```python
from build123d import *

# Parameters (mm, degrees)
SKETCH2_R               = 3
CUT_EXTRUDE2_DEPTH      = 21
CUT_EXTRUDE2_DEPTH_BACK = 1
SKETCH3_R               = 5.5
CUT_EXTRUDE3_DEPTH      = 11
CUT_EXTRUDE4_REACH      = 16.5
SKETCH4_R               = 1.25
CHAMFER1_SIZE           = 1


with BuildPart() as part:
    # Sketch1 → Revolve1 (revolve)
    with BuildSketch(Plane.XY):
        Polygon((27.5, 0), (27.5, 20), (25, 20), (25, 13.5), (12, 13.5), (12, 20), (0, 20), (0, 5.5), (22.4, 5.5), (22.4, 0), align=None)
    revolve(axis=Axis((0, -626.687351978, 0), (0, 1, 0)))

    # Sketch2 → Cut-Extrude2 (cut, two sides)
    with BuildSketch(Plane(origin=(0, 0, 0), x_dir=(1, 0, 0), z_dir=(0, 1, 0))) as cut_extrude2_sk:
        with Locations((-14.142135624, 14.142135624)):
            Circle(SKETCH2_R)
        with Locations((14.142135624, 14.142135624)):
            Circle(SKETCH2_R)
        with Locations((14.142135624, -14.142135624)):
            Circle(SKETCH2_R)
        with Locations((-14.142135624, -14.142135624)):
            Circle(SKETCH2_R)
    extrude(amount=CUT_EXTRUDE2_DEPTH, mode=Mode.SUBTRACT)
    extrude(cut_extrude2_sk.sketch, amount=-CUT_EXTRUDE2_DEPTH_BACK, mode=Mode.SUBTRACT)

    # Sketch3 → Cut-Extrude3 (cut)
    with BuildSketch(Plane.XZ):
        with Locations((-14.142135624, 14.142135624)):
            Circle(SKETCH3_R)
        with Locations((14.142135624, 14.142135624)):
            Circle(SKETCH3_R)
        with Locations((14.142135624, -14.142135624)):
            Circle(SKETCH3_R)
        with Locations((-14.142135624, -14.142135624)):
            Circle(SKETCH3_R)
    extrude(amount=-CUT_EXTRUDE3_DEPTH, mode=Mode.SUBTRACT)

    # Sketch4 → Cut-Extrude4 (cut, up to next)
    with BuildSketch(Plane.XZ.offset(-5.5), mode=Mode.PRIVATE) as cut_extrude4_sk1:
        with Locations((0, 20)):
            Circle(SKETCH4_R)
    cut_extrude4_tool1 = extrude(cut_extrude4_sk1.sketch, amount=-CUT_EXTRUDE4_REACH, mode=Mode.PRIVATE) & part.part
    add(cut_extrude4_tool1.solids().sort_by_distance((0, 5.5, 20))[0], mode=Mode.SUBTRACT)
    # Sketch4 → Cut-Extrude4 (cut, up to next)
    with BuildSketch(Plane.XZ.offset(-5.5), mode=Mode.PRIVATE) as cut_extrude4_sk2:
        with Locations((-20, 0)):
            Circle(SKETCH4_R)
    cut_extrude4_tool2 = extrude(cut_extrude4_sk2.sketch, amount=-CUT_EXTRUDE4_REACH, mode=Mode.PRIVATE) & part.part
    add(cut_extrude4_tool2.solids().sort_by_distance((-20, 5.5, 0))[0], mode=Mode.SUBTRACT)
    # Sketch4 → Cut-Extrude4 (cut, up to next)
    with BuildSketch(Plane.XZ.offset(-5.5), mode=Mode.PRIVATE) as cut_extrude4_sk3:
        with Locations((0, -20)):
            Circle(SKETCH4_R)
    cut_extrude4_tool3 = extrude(cut_extrude4_sk3.sketch, amount=-CUT_EXTRUDE4_REACH, mode=Mode.PRIVATE) & part.part
    add(cut_extrude4_tool3.solids().sort_by_distance((0, 5.5, -20))[0], mode=Mode.SUBTRACT)
    # Sketch4 → Cut-Extrude4 (cut, up to next)
    with BuildSketch(Plane.XZ.offset(-5.5), mode=Mode.PRIVATE) as cut_extrude4_sk4:
        with Locations((20, 0)):
            Circle(SKETCH4_R)
    cut_extrude4_tool4 = extrude(cut_extrude4_sk4.sketch, amount=-CUT_EXTRUDE4_REACH, mode=Mode.PRIVATE) & part.part
    add(cut_extrude4_tool4.solids().sort_by_distance((20, 5.5, 0))[0], mode=Mode.SUBTRACT)

    # Chamfer1
    chamfer1_edges = [part.edges().sort_by_distance(p)[0] for p in [
        (-12, 20, 0),
        (-27.5, 0, 0),
        (-27.5, 20, 0),
    ]]
    chamfer(chamfer1_edges, length=CHAMFER1_SIZE)


solid = part.part
```
Geometry: final body of the model. Coordinates: model frame, mm. A direction names the side the tool comes from. Round coordinates to 2 decimals unless told otherwise and drop trailing zeros. Write each loop counter-clockwise with the first axis right and the second up, starting at its lowest first coordinate (ties: lowest second). Pieces come first, ordered by that corner, then holes. Notation, with made-up numbers: (-14, -33.5) -> (-9, -33.5) arc R7 ccw to (-9, -22.5) -> close; hole circle Ø4 at (12.5, 34). An arc over 180 degrees is marked (long way). Use CSV: the item, a comma, the result in double quotes. Start each with the question number.
Q1. Line query: L1, parallel to X at y = 18.5, z = 0; L2, parallel to X at y = 16.5, z = -9; L3, parallel to Z at x = -8, y = 19. Output: solid intervals per line, ascending.
Q2. Section A-A (x = 0). Give the number of separate pieces and of enclosed holes in the cut face, plus the area to 3 significant figures.
Q3. Section C-C (y = 18). Return loops of the section in (x, z), plus the area to 3 significant figures.
Q4. Reachability of faces 1 (the face through (-18.845, 9.444, -0.479)), 2 (the face through (-18.5, 6.6, -17.5)) from +Z, -Z, +X, -X, +Y, -Y: full face, straight path, thin tool, end or side. Return the list, or none.
Q5. Pull-direction query (Z, two-part tool) for faces 3 (the face through (20, 20, -16)), 4 (the face through (-5.961, 10.126, 26.846)), 5 (the face through (-6, 13.5, 11)); classes: pulls with the +Z half, pulls with the -Z half, needs draft (parallel to the pull), parting line crosses it, or undercut.
Q6. Section D-D (y = 3). Return loops of the section in (x, z).
Q7. First-contact query: pin 1 Ø5.5 at (x, z) = (16.5, -13.5) entering from -Y; pin 2 Ø2 at (x, z) = (15.5, 4.5) entering from -Y; pin 3 Ø4 at (x, z) = (0, -20) entering from +Y. Flat tips, straight axial feed; report the tip coordinate or a pass-through.
Result sheet:
1,L1,"-27.5 to -25, -12 to 12, 25 to 27.5"
1,L2,"-25.99 to -23.32, -7.94 to 7.94, 23.32 to 25.99"
1,L3,"-26.31 to -23.69, -8.94 to 8.94, 23.69 to 26.31"
2,separate pieces,"3"
2,enclosed holes,"0"
2,area,"642 mm²"
3,outline,"circle Ø55 at (0, 0); circle Ø24 at (0, 0); hole circle Ø50 at (0, 0)"
3,area,"865 mm²"
4,face 1,"+Y, -Y"
4,face 2,"-Y"
5,face 3,"needs draft"
5,face 4,"parting line crosses it"
5,face 5,"undercut"
6,outline,"circle Ø55 at (0, 0); hole (-19.08, -11.73) arc R5.5 ccw to (-11.73, -19.08) arc R22.4 ccw to (11.73, -19.08) arc R5.5 ccw to (19.08, -11.73) arc R22.4 ccw to (19.08, 11.73) arc R5.5 ccw to (11.73, 19.08) arc R22.4 ccw to (-11.73, 19.08) arc R5.5 ccw to (-19.08, 11.73) arc R22.4 ccw to start"
7,pin 1,"y = 11"
7,pin 2,"y = 5.5"
7,pin 3,"y = 13.5"
